Verification items for the finished model (mm, model axes). Face numbers are marked on the shaded views. A direction names the side the tool comes from. Round coordinates to 2 decimals unless told otherwise and drop trailing zeros. Order: outer loops, then holes, each group sorted by start corner. A loop starts at its lowest first (then second) coordinate and runs counter-clockwise, first axis right, second up. Notation, with made-up numbers: M -4,46 L 54,46 A15 cw 54,56 Z; hole C 67,-9.75 d6. An arc over 180 degrees is marked long. Use one line per item in the form item = value. Start each with the question number.
Item 1: Thickness scan on probe 1 along X at (y, z) = (0, 2.5); probe 2 along X at (y, z) = (-0.5, 6.25); probe 3 along Z at (x, y) = (1.75, 1.25). Record the ranges inside material, lowest first. Write a range as [from, to].
Item 2: Go/stop test with flat-tipped pins: pin 1 Ø2 at (y, z) = (2, -0.5) entering from -X; pin 2 Ø1 at (x, z) = (0.5, 5) entering from +Y; pin 3 Ø3 at (x, z) = (-0.5, 2.5) entering from -Y. Record where each tip stops, or that it passes through.
Item 3: Tool access check on the marked faces 1 and 2. Record the directions out of +Z, -Z, +X, -X, +Y, -Y that give a thin tool (end or side, any length) a straight path to the whole face; none if there is none.
Item 4: Cross-section at A-A on z = 1.75. Enter the section's corners in (x, y), then the cut area to 3 significant figures.
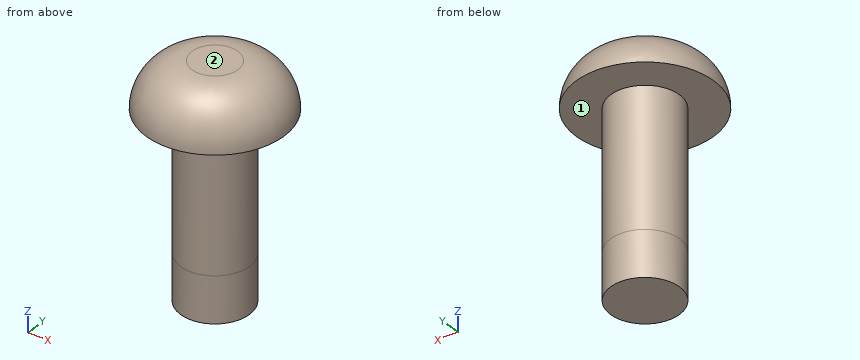
Autodesk Inventor part; units mm, degrees
ref_plane "YZ Plane" through (0, 0, 0) normal (1, 0, 0) x (0, 1, 0)
ref_plane "XZ Plane" through (0, 0, 0) normal (0, 1, 0) x (-1, 0, 0)
ref_plane "XY Plane" through (0, 0, 0) normal (0, 0, 1) x (1, 0, 0)
sketch "スケッチ1" plane through (0, 0, 0) normal (0, 0, 1) x (1, 0, 0)
  circle A0 centre (0, 0) radius 1.5
  dimension "d0" = 3
extrude "押し出し1" add sketch "スケッチ1" along normal blind 6
sketch "スケッチ2" plane through (0, 0, 6) normal (0, 0, 1) x (1, 0, 0)
  circle A0 centre (0, 0) radius 1.5
  circle A1 centre (0, 0) radius 3
  dimension "d3" = 6
extrude "押し出し2" add sketch "スケッチ2" along normal blind 2 contours A0 | A1
fillet "フィレット1" radius 2 1 edges at (-3, 0, 8)
thread "ねじ1"
sketch "スケッチ3" plane through (0, 0, 0) normal (0, 0, -1) x (-1, 0, 0)
  circle A0 centre (0, 0) radius 1.5
extrude "押し出し3" add sketch "スケッチ3" along normal blind 2
properties part number "SB　8mmなべネジ" material "Steel, Mild"
Output values:
q1.probe_1 = [-1.5, 1.5]
q1.probe_2 = [-2.94, 2.94]
q1.probe_3 = [6, 7.64]
q2.pin_1 = -1.12
q2.pin_2 = 1.5
q2.pin_3 = -1.5
q3.face_1 = -Z
q3.face_2 = +Z, +X, -X, +Y, -Y
q4.outline = C 0,0 d3
q4.area = 7.07 mm2
